For this review, take the finished solid that the model builds, in its own axes (mm). A direction names the side the tool comes from. Coordinates: 2 decimals unless noted, no trailing zeros. Order: outer loops, then holes, each group sorted by start corner. A loop starts at its lowest first (then second) coordinate and runs counter-clockwise, first axis right, second up. Notation, with made-up numbers: M 88.25,-23.5 L 97.25,-23.5 A29 ccw 97.25,-0.5 Z; hole C 28.5,67.25 d7. An arc over 180 degrees is marked long. Use one line per item in the form item = value. Start each with the question number.
```python
from build123d import *

# Parameters (mm, degrees)
SKETCH1_W           = 35
SKETCH1_H           = 35
BOSS_EXTRUDE1_DEPTH = 8
SKETCH2_W           = 5
SKETCH2_H           = 7
SKETCH2_W_2         = 7
SKETCH2_H_2         = 5
SKETCH2_R           = 1.5
CUT_EXTRUDE1_DEPTH  = 9
SKETCH2_5_R         = 4
SKETCH2_5_R_2       = 1.5
CUT_EXTRUDE2_DEPTH  = 4
SKETCH2_7_R         = 5
SKETCH2_7_R_2       = 2.5
BOSS_EXTRUDE2_DEPTH = 150
SKETCH3_W           = 18
SKETCH3_H           = 18
BOSS_EXTRUDE3_DEPTH = 4
FILLET1_R           = 5


with BuildPart() as part:
    # Sketch1 → Boss-Extrude1 (new body)
    with BuildSketch(Plane(origin=(0, 0, 0), x_dir=(1, 0, 0), z_dir=(0, 1, 0))):
        with Locations((17.5, 17.5)):
            Rectangle(SKETCH1_W, SKETCH1_H)
    extrude(amount=BOSS_EXTRUDE1_DEPTH)

    # Sketch2 → Cut-Extrude1 (cut, through all)
    with BuildSketch(Plane.XZ):
        with Locations((32.5, -21.5)):
            Rectangle(SKETCH2_W, SKETCH2_H)
        with Locations((13.5, -32.5)):
            Rectangle(SKETCH2_W_2, SKETCH2_H_2)
        with Locations((2.5, -13.5)):
            Rectangle(SKETCH2_W, SKETCH2_H)
        with Locations((21.5, -2.5)):
            Rectangle(SKETCH2_W_2, SKETCH2_H_2)
        with Locations((11, -11)):
            Circle(SKETCH2_R)
        with Locations((24, -11)):
            Circle(SKETCH2_R)
        with Locations((11, -24)):
            Circle(SKETCH2_R)
        with Locations((24, -24)):
            Circle(SKETCH2_R)
    extrude(amount=-CUT_EXTRUDE1_DEPTH, mode=Mode.SUBTRACT)

    # Sketch2_5 → Cut-Extrude2 (cut)
    with BuildSketch(Plane.XZ):
        with Locations((6, -29)):
            Circle(SKETCH2_5_R)
        with Locations((29, -6)):
            Circle(SKETCH2_5_R)
        with Locations((11, -11)):
            Circle(SKETCH2_5_R_2)
    extrude(amount=-CUT_EXTRUDE2_DEPTH, mode=Mode.SUBTRACT)

    # Sketch2_7 → Boss-Extrude2 (add)
    with BuildSketch(Plane.XZ):
        with Locations((17.5, -17.5)):
            Circle(SKETCH2_7_R)
        with Locations((29, -29)):
            Circle(SKETCH2_7_R_2)
        with Locations((6, -6)):
            Circle(SKETCH2_7_R_2)
    extrude(amount=BOSS_EXTRUDE2_DEPTH)

    # Sketch3 → Boss-Extrude3 (add)
    with BuildSketch(Plane(origin=(0, -150, 0), x_dir=(-1, 0, 0), z_dir=(0, -1, 0))):
        with Locations((-17.5, 17.5)):
            Rectangle(SKETCH3_W, SKETCH3_H)
    extrude(amount=BOSS_EXTRUDE3_DEPTH)

    # Fillet1
    fillet1_edges = [part.edges().sort_by_distance(p)[0] for p in [
        (0, 4, -35),
        (35, 4, -35),
        (35, 4, 0),
        (0, 4, 0),
    ]]
    fillet(fillet1_edges, radius=FILLET1_R)


solid = part.part
```
1. Consider section B-B, the plane x = 14. Write out the cut boundary in (y, z), plus the area to 3 significant figures.
2. To check wall thickness, follow line 1 (Z direction, x = 11, y = 2.5); line 2 (Z direction, x = 24, y = 2.25); line 3 (Y direction, x = 13, z = -26). State the ranges of each line that lie inside material, in increasing order.
3. Consider section A-A, the plane y = -78.5. Write out the cut boundary in (x, z).
4. Tool access review of faces 1 (the cylindrical face through (16.42, -73.95, -22.38)), 2 (the flat face through (21, 4, -5)), 3 (the flat face through (13, 4, -30)): name each direction out of +Z, -Z, +X, -X, +Y, -Y from which nothing blocks a thin tool from reaching the whole face with its end or side.
5. For pin 1 Ø12 at (x, y) = (13, -30) entering from -Z; pin 2 Ø1.5 at (y, z) = (-80.5, -21) entering from -X; pin 3 Ø2.5 at (y, z) = (4, -31.5) entering from -X; pin 4 Ø5.5 at (x, y) = (3, 3) entering from +Z, all flat-tipped, find the tip position at first contact; note any pin that passes through.
6. The part is to be moulded in two halves that separate along X. For faces 4 (the cylindrical face through (33, 4, -34)), 5 (the flat face through (23, 4, -35)), 6 (the flat face through (18, 4, -3)), say which applies: pulls with the +X half, pulls with the -X half, needs draft (parallel to the pull), parting line crosses it, or undercut.
Answers follow:
q1.outline = M -154,-26.5 L -150,-26.5 L -150,-21.07 L 0,-21.07 L 0,-30 L 8,-30 L 8,0 L 0,0 L 0,-13.93 L -150,-13.93 L -150,-8.5 L -154,-8.5 Z
q1.area = 1,380 mm²
q2.line_1 = -30 to -25.5, -22.5 to -12.5, -9.5 to 0
q2.line_2 = -35 to -25.5, -22.5 to -12.5, -9.5 to -5
q2.line_3 = -154 to -150, 0 to 8
q3.outline = C 6,-6 d5; C 17.5,-17.5 d10; C 29,-29 d5
q4.face_1 = none
q4.face_2 = +Z, +Y, -Y
q4.face_3 = -Z, +Y, -Y
q5.pin_1 = -22.5
q5.pin_2 = 13.32
q5.pin_3 = 0.01
q5.pin_4 = 0
q6.face_4 = pulls with the +X half
q6.face_5 = needs draft
q6.face_6 = undercut
